```python
from build123d import *

# Parameters (mm, degrees)
F1_DEPTH = 20


with BuildPart() as f1:
    # F0 (on Top) → F1 (new body)
    with BuildSketch(Plane.XY):
        with BuildLine():
            ThreePointArc((-5.697157, 20.32), (5.021446, 20.721446), (10.5, 11.5))
            Line((10.5, 11.5), (10.5, -11.5))
            ThreePointArc((10.5, -11.5), (5.021446, -20.721446), (-5.697157, -20.32))
            ThreePointArc((-5.697157, -20.32), (-8.46233, -20.914827), (-7.867503, -23.68))
            ThreePointArc((-7.867503, -23.68), (6.934378, -24.234378), (14.5, -11.5))
            Line((14.5, -11.5), (14.5, 11.5))
            ThreePointArc((14.5, 11.5), (6.934378, 24.234378), (-7.867503, 23.68))
            ThreePointArc((-7.867503, 23.68), (-8.46233, 20.914827), (-5.697157, 20.32))
        make_face()
    extrude(amount=F1_DEPTH)


solid = f1.part
```
Verification items for the finished model (mm, model axes). A direction names the side the tool comes from. Round coordinates to 2 decimals unless told otherwise and drop trailing zeros. Write each loop counter-clockwise with the first axis right and the second up, starting at its lowest first coordinate (ties: lowest second). Pieces come first, ordered by that corner, then holes.
1. Gauge pin test, flat ends, axial feed: P1, Ø12, axis at y = -1, z = 6.5, coming from the -X side; P2, Ø1, axis at y = 20, z = 11, coming from the +X side; P3, Ø1.5, axis at x = 1.5, z = 12.5, coming from the -Y side; P4, Ø4, axis at x = 4, y = 17.5, coming from the +Z side. Record the tip position at first contact, or that the pin passes through.
2. Section check A-A on z = 8. Enter the section's corners in (x, y).
3. Section check C-C on y = 1.5. Enter the section's corners in (x, z).
4. Section check B-B on x = 3. Enter the section's corners in (y, z), plus the area to 3 significant figures.
5. Access from +Z, -Z, +X, -X, +Y, -Y to the whole of each face (thin tool, end or side, straight path). Record for faces 5 (the flat face through (10.5, 0, 10)), 6 (the flat face through (11, 2, 20)), 7 (the cylindrical face through (5.159, -20.645, 9.86)).
6. Scan lines: L1, parallel to X at y = -4.5, z = 15; L2, parallel to Y at x = 1, z = 7; L3, parallel to Y at x = 4, z = 9.25. Record each from-to range of solid material in increasing order.
7. Section check D-D on x = 10. Enter the section's corners in (y, z).
8. Draft check along X on faces 1 (the flat face through (11, 2, 0)), 2 (the cylindrical face through (-8.486, 20.952, 9.86)), 3 (the cylindrical face through (7.12, 24.13, 9.86)), 4 (the cylindrical face through (4.882, 20.796, 9.86)). Enter one of: +X half, -X half, draft (parallel to the pull), parting line (faces both ways), or undercut.
Answer:
1. P1: stops at x = 10.5
1. P2: stops at x = 12.09
1. P3: stops at y = -25.98
1. P4: passes through
2. outline: (-7.87, -23.68) arc R14.5 ccw to (14.5, -11.5) - (14.5, 11.5) arc R14.5 ccw to (-7.87, 23.68) arc R2 ccw to (-5.7, 20.32) arc R10.5 cw to (10.5, 11.5) - (10.5, -11.5) arc R10.5 cw to (-5.7, -20.32) arc R2 ccw to start
3. outline: (10.5, 0) - (14.5, 0) - (14.5, 20) - (10.5, 20) - close
4. outline: (-25.69, 0) - (-21.56, 0) - (-21.56, 20) - (-25.69, 20) - close; (21.56, 0) - (25.69, 0) - (25.69, 20) - (21.56, 20) - close
4. area: 165 mm2
5. face 5: +Z, -Z, -X
5. face 6: +Z, +X, -X, +Y, -Y
5. face 7: +Z, -Z
6. L1: x = 10.5 to 14.5
6. L2: y = -25.97 to -21.95, 21.95 to 25.97
6. L3: y = -25.44 to -21.21, 21.21 to 25.44
7. outline: (-22, 0) - (-14.7, 0) - (-14.7, 20) - (-22, 20) - close; (14.7, 0) - (22, 0) - (22, 20) - (14.7, 20) - close
8. face 1: draft
8. face 2: undercut
8. face 3: parting line
8. face 4: undercut
